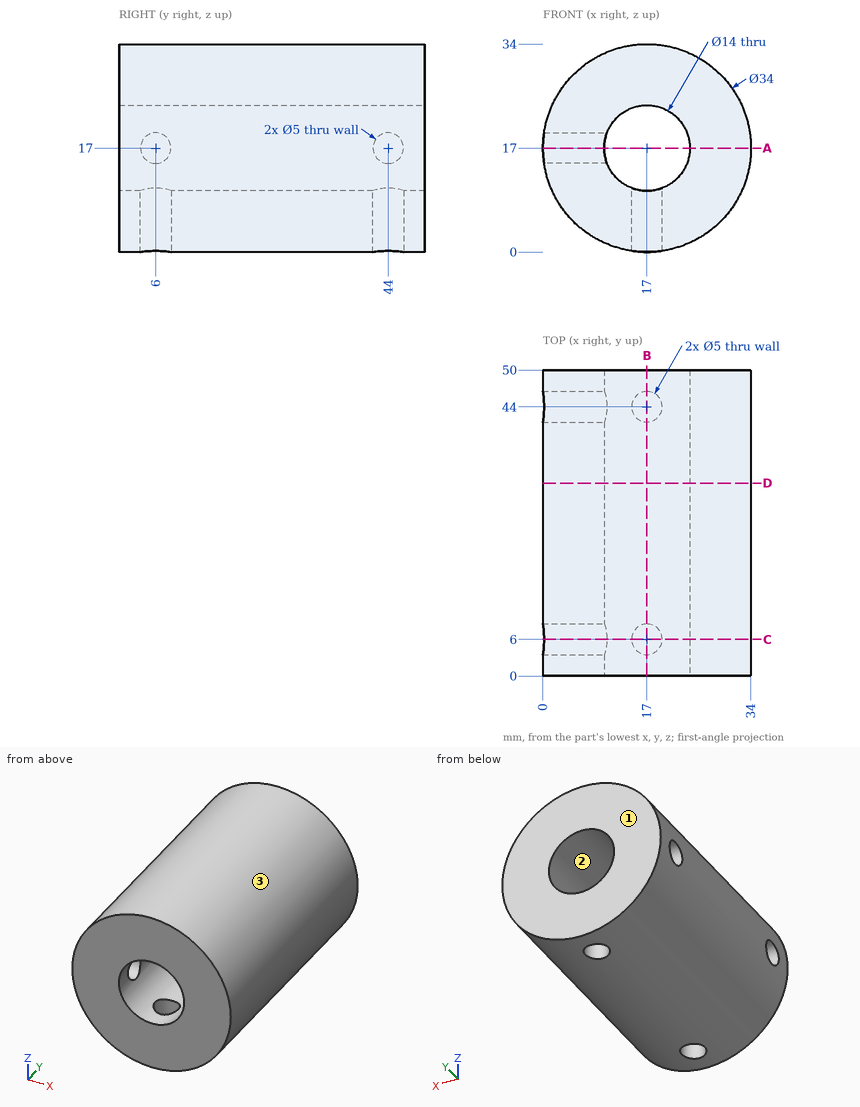
The drawing under review shows one solid part. Ordinate dimensions are in mm from its lowest x, y, z. Coordinates: 2 decimals unless noted, no trailing zeros. Order: outer loops, then holes, each group sorted by start corner. A loop starts at its lowest first (then second) coordinate and runs counter-clockwise, first axis right, second up. Notation, with made-up numbers: (-26.75, -29) -> (27.25, -29) arc R36 cw to (27.25, 7) -> close; hole circle Ø9 at (48.5, 39.5). An arc over 180 degrees is marked (long way). Answer in a Markdown table with one row per item.
(1) Consider section B-B (x = 17). Write out the cut boundary in (y, z), plus the area to 3 significant figures.
Answers:
| item | result |
|---|---|
| outline | (0, 0) -> (3.5, 0) -> (3.5, 10) -> (0, 10) -> close; (0, 24) -> (50, 24) -> (50, 34) -> (0, 34) -> close; (8.5, 0) -> (41.5, 0) -> (41.5, 10) -> (8.5, 10) -> close; (46.5, 0) -> (50, 0) -> (50, 10) -> (46.5, 10) -> close |
| area | 900 mm² |
(2) Insertion check: pin 1 (5 mm diameter, centred on x = 26, y = 41, fed in from -Z); pin 2 (1.5 mm diameter, centred on y = 26, z = 12, fed in from -X); pin 3 (4 mm diameter, centred on y = 19.5, z = 21.5, fed in from +X). Each pin has a flat end and moves straight along its axis. Give the tip position at first contact, or say it passes through.
Answers:
| item | result |
|---|---|
| pin 1 | z = 1.29 |
| pin 2 | x = 0.54 |
| pin 3 | x = 33.82 |
(3) Consider section D-D (y = 31.5). Write out the cut boundary in (x, z).
Answers:
| item | result |
|---|---|
| outline | circle Ø34 at (17, 17); hole circle Ø14 at (17, 17) |
(4) Wall thickness on line 1 along Y through (x, z) = (6.5, 17); line 2 along X through (y, z) = (28, 17); line 3 along X through (y, z) = (42, 11): over which ranges is each line inside the solid? List them lowest first.
Answers:
| item | result |
|---|---|
| line 1 | 0 to 3.5, 8.5 to 41.5, 46.5 to 50 |
| line 2 | 0 to 10, 24 to 34 |
| line 3 | 1.09 to 13.39, 20.61 to 32.91 |
(5) The part is to be moulded in two halves that separate along Z. For the marked faces 1, 2 and 3, say which applies: +Z half, -Z half, draft (parallel to the pull), parting line (faces both ways), or undercut.
Answers:
| item | result |
|---|---|
| face 1 | draft |
| face 2 | undercut |
| face 3 | parting line |
(6) Consider section A-A (z = 17). Write out the cut boundary in (x, y), plus the area to 3 significant figures.
Answers:
| item | result |
|---|---|
| outline | (0, 0) -> (10, 0) -> (10, 3.5) -> (0, 3.5) -> close; (0, 8.5) -> (10, 8.5) -> (10, 41.5) -> (0, 41.5) -> close; (0, 46.5) -> (10, 46.5) -> (10, 50) -> (0, 50) -> close; (24, 0) -> (34, 0) -> (34, 50) -> (24, 50) -> close |
| area | 900 mm² |
(7) Consider section C-C (y = 6). Write out the cut boundary in (x, z), plus the area to 3 significant figures.
Answers:
| item | result |
|---|---|
| outline | (0.18, 14.5) arc R17 ccw to (14.5, 0.18) -> (14.5, 10.46) arc R7 cw to (10.46, 14.5) -> close; (0.18, 19.5) -> (10.46, 19.5) arc R7 cw (long way) to (19.5, 10.46) -> (19.5, 0.18) arc R17 ccw (long way) to start |
| area | 653 mm² |
